Geometry: final body of the model. Coordinates: model frame, mm. A direction names the side the tool comes from. Give positions to 0.01 mm unless a question says otherwise; leave off trailing zeros. Write each loop counter-clockwise with the first axis right and the second up, starting at its lowest first coordinate (ties: lowest second). Pieces come first, ordered by that corner, then holes. Notation, with made-up numbers: (-14.75, -26.5) -> (35.25, -26.5) arc R27 ccw to (35.25, -7.5) -> close; hole circle Ø10 at (-7, 20.5). An arc over 180 degrees is marked (long way). Answer as a JSON object with one key per item and string values. Group by question number.
(1) Section query A-A on z = 0.6. Output: boundary loops of the cut face in (x, y), plus the area to 3 significant figures.
(2) Material intervals for probe 1 along Y at (x, z) = (53.75, 0.2); probe 2 along Y at (x, z) = (56.5, 0.45); probe 3 along X at (y, z) = (41, 0.4), sorted ascending.
(3) Set-up query: faces 1 (the face through (58.347, 18.7, 0.4)), 2 (the face through (54.3, 38.25, 0.44)), 3 (the face through (54.9, 15.1, 0.4)). Return all of +Z, -Z, +X, -X, +Y, -Y with unobstructed straight access to the full face (end or side cutting, diameter ignored); none if empty.
(4) Contact query for a flat-ended pin moving along its axis: pin 1 Ø1.5 at (x, y) = (55.6, 41.34) entering from -Z. Output: stop coordinate, or through.
(5) Section query C-C on y = 55. Output: boundary loops of the cut face in (x, z).
(6) Section query B-B on y = 19.5. Output: boundary loops of the cut face in (x, z).
(7) Draft query along X for faces 4 (the face through (52.31, 54.62, 0.44)), 5 (the face through (55.46, 26.03, 0.44)), 6 (the face through (56, 38, 0)). Return one class per face: +X half, -X half, draft (parallel to the pull), parting line (faces both ways), or undercut.
(8) Section query D-D on y = 45. Output: boundary loops of the cut face in (x, z), plus the area to 3 significant figures.
from build123d import *

# Parameters (mm, degrees)
SKETCH1_R           = 1.27
BOSS_EXTRUDE3_DEPTH = 0.889
SKETCH3_R           = 2.032
CUT_EXTRUDE1_DEPTH  = 1.889
CUT_EXTRUDE2_DEPTH  = 24.373709


with BuildPart() as part:
    # Sketch1 → Boss-Extrude3 (new body)
    with BuildSketch(Plane.XY):
        with BuildLine():
            Line((53.882826418, 59.421700713), (56.230021181, 46.213700713))
            ThreePointArc((56.230021181, 46.213700713), (56.248351323, 44.442871919), (57.525920997, 43.216500713))
            Line((57.525920997, 43.216500713), (59.870620113, 20.102500713))
            Line((59.870620113, 20.102500713), (58.346620113, 20.102500713))
            Line((58.346620113, 20.102500713), (58.346620113, 17.308500713))
            ThreePointArc((58.346620113, 17.308500713), (54.868586202, 15.099346005), (51.475082329, 17.436270454))
            Line((51.475082329, 17.436270454), (51.475082329, 24.802270454))
            ThreePointArc((51.475082329, 24.802270454), (52.66510076, 25.100716041), (53.529437672, 25.971425715))
            ThreePointArc((53.529437672, 25.971425715), (55.487269989, 26.051421604), (56.18260068, 27.883366459))
            Line((56.18260068, 27.883366459), (55.54760068, 37.433766459))
            Line((55.54760068, 37.433766459), (53.019584786, 39.084766459))
            ThreePointArc((53.019584786, 39.084766459), (52.015147123, 44.373161392), (51.741430513, 49.749135277))
            ThreePointArc((51.741430513, 49.749135277), (52.3260698, 54.693025851), (53.882826418, 59.421700713))
        make_face()
        with Locations((55.59840068, 41.336900713)):
            Circle(SKETCH1_R, mode=Mode.SUBTRACT)
        with Locations((54.27760068, 23.912500713)):
            Circle(SKETCH1_R, mode=Mode.SUBTRACT)
    extrude(amount=BOSS_EXTRUDE3_DEPTH)

    # Sketch3 → Cut-Extrude1 (cut, through all)
    with BuildSketch(Plane.XY.offset(0.889)):
        with Locations((54.93800068, 18.832500713)):
            Circle(SKETCH3_R)
    extrude(amount=-CUT_EXTRUDE1_DEPTH, mode=Mode.SUBTRACT)

    # Sketch4 → Cut-Extrude2 (cut)
    with BuildSketch(Plane(origin=(-10.504426242, 59.109905984, 0), x_dir=(0.984573992, 0.174968725, 0), z_dir=(-0.174968725, 0.984573992, 0))):
        Polygon((63.448568698, 0), (63.448568698, -0.889), (62.935304309, -0.889), align=None)
    extrude(amount=-CUT_EXTRUDE2_DEPTH, mode=Mode.SUBTRACT)


solid = part.part
Answer list:
{
 "1": {"outline": "(51.48, 17.44) arc R3.73 ccw to (58.35, 17.31) -> (58.35, 20.1) -> (59.87, 20.1) -> (57.53, 43.22) arc R2.29 cw to (56.23, 46.21) -> (55.89, 46.15) -> (53.63, 58.84) arc R24.89 ccw to (51.74, 49.75) arc R39.37 ccw to (53.02, 39.08) -> (55.55, 37.43) -> (56.18, 27.88) arc R1.78 cw to (53.53, 25.97) arc R2.29 cw to (51.48, 24.8) -> close; hole circle Ø4.06 at (54.94, 18.83); hole circle Ø2.54 at (54.28, 23.91); hole circle Ø2.54 at (55.6, 41.34)", "area": "157 mm2"},
 "2": {"probe 1": "15.29 to 17.18, 20.48 to 22.76, 25.07 to 25.86, 38.61 to 59.12", "probe 2": "15.44 to 17.53, 20.13 to 40.44, 42.23 to 44", "probe 3": "52.57 to 54.37, 56.82 to 57.75"},
 "3": {"face 1": "+Z, -Z, +X, -Y", "face 2": "+Z, -Z, -X", "face 3": "+Z, -Z, -Y"},
 "4": {"pin 1": "through"},
 "5": {"outline": "(52.4, 0) -> (54.67, 0) -> (54.15, 0.89) -> (52.4, 0.89) -> close"},
 "6": {"outline": "(51.48, 0) -> (53.02, 0) -> (53.02, 0.89) -> (51.48, 0.89) -> close; (56.86, 0) -> (58.35, 0) -> (58.35, 0.89) -> (56.86, 0.89) -> close"},
 "7": {"face 4": "-X half", "face 5": "undercut", "face 6": "draft"},
 "8": {"outline": "(51.95, 0) -> (56.09, 0) -> (56.09, 0.89) -> (51.95, 0.89) -> close", "area": "3.68 mm2"}
}
